```python
from build123d import *

# Parameters (mm, degrees)
SKETCH1_R              = 5.08
BOSS_EXTRUDE1_DEPTH    = 6.35
F_10_32_TAPPED_HOLE1_D = 4.826
SKETCH7_R              = 8.73125
CUT_EXTRUDE1_DEPTH     = 7.35
SKETCH8_R              = 6.35
CUT_EXTRUDE2_DEPTH     = 7.35
FILLET1_R              = 25.4
FILLET2_R              = 6.35
F_4_40_TAPPED_HOLE1_D  = 2.2606


with BuildPart() as part:
    # Sketch1 → Boss-Extrude1 (new body)
    with BuildSketch(Plane(origin=(0, 0, 0), x_dir=(1, 0, 0), z_dir=(0, 1, 0))):
        with Locations((0, -15.08125)):
            Circle(SKETCH1_R)
        with BuildLine():
            Line((1.984375, -15.750488274), (-48.417187476, -22.100488274))
            ThreePointArc((-48.417187476, -22.100488274), (-66.152050749, -8.334375), (-52.385937476, 9.400488274))
            Line((-52.385937476, 9.400488274), (-1.984375, 15.750488274))
            ThreePointArc((-1.984375, 15.750488274), (15.750488274, 1.984375), (1.984375, -15.750488274))
        make_face()
        with BuildLine():
            Line((1.984375, 15.750488274), (52.385937476, 9.400488274))
            ThreePointArc((52.385937476, 9.400488274), (66.152050749, -8.334375), (48.417187476, -22.100488274))
            Line((48.417187476, -22.100488274), (-1.984375, -15.750488274))
            ThreePointArc((-1.984375, -15.750488274), (-15.750488274, 1.984375), (1.984375, 15.750488274))
        make_face()
    extrude(amount=BOSS_EXTRUDE1_DEPTH)

    # #10-32 Tapped Hole1 (through all)
    with Locations(Plane(origin=(0, 6.35, 0), x_dir=(1, 0, 0), z_dir=(0, 1, 0))):
        with Locations((-50.401562476, -6.35), (50.401562476, -6.35)):
            Hole(F_10_32_TAPPED_HOLE1_D / 2)

    # Sketch7 → Cut-Extrude1 (cut, through all)
    with BuildSketch(Plane(origin=(0, 6.35, 0), x_dir=(1, 0, 0), z_dir=(0, 1, 0))):
        Circle(SKETCH7_R)
    extrude(amount=-CUT_EXTRUDE1_DEPTH, mode=Mode.SUBTRACT)

    # Sketch8 → Cut-Extrude2 (cut, through all)
    with BuildSketch(Plane(origin=(0, 6.35, 0), x_dir=(1, 0, 0), z_dir=(0, 1, 0))):
        with Locations((-38.1, 12.7)):
            Circle(SKETCH8_R)
        with Locations((38.1, 12.7)):
            Circle(SKETCH8_R)
    extrude(amount=-CUT_EXTRUDE2_DEPTH, mode=Mode.SUBTRACT)

    # Fillet1
    fillet1_edges = [part.edges().sort_by_distance(p)[0] for p in [
        (-4.844257487, 3.175, 16.6108151),
        (4.844257487, 3.175, 16.6108151),
    ]]
    fillet(fillet1_edges, radius=FILLET1_R)

    # Fillet2
    fillet2_edges = [part.edges().sort_by_distance(p)[0] for p in [
        (-31.789208912, 3.175, -11.995432159),
        (-44.038818433, 3.175, -10.452126424),
        (31.789208912, 3.175, -11.995432159),
        (44.038818433, 3.175, -10.452126424),
    ]]
    fillet(fillet2_edges, radius=FILLET2_R)

    # #4-40 Tapped Hole1 (through all)
    with Locations(Plane(origin=(0, 6.35, 0), x_dir=(1, 0, 0), z_dir=(0, 1, 0))):
        with Locations((-15.08125, 0), (15.08125, 0), (0, -15.08125)):
            Hole(F_4_40_TAPPED_HOLE1_D / 2)


solid = part.part
```
Read the model definition and answer for the solid it produces. Units are mm, in the model's axes. A direction names the side the tool comes from. Coordinates: 2 decimals unless noted, no trailing zeros. Loops run counter-clockwise (first coordinate to the right, second up) from the corner with the lowest first, then second, coordinate; pieces in that order, holes last.
(1) A tool of negligible diameter and unlimited length cuts with its end or side. For faces 1 (the face through (-31.551, 3.131, 19.976)), 2 (the face through (-47.99, 3.13, 6.24)), from which of +Z, -Z, +X, -X, +Y, -Y can it reach the whole face along a straight path? Write none if from no direction.
Solution:
face 1: +Z, +Y, -Y
face 2: +Y, -Y
(2) The part is cut by section D-D (z = 6.35). Determine the outline of the cut face in (x, y), and give its area (3 significant figures).
Solution:
outline: (-66.28, 0) - (-52.81, 0) - (-52.81, 6.35) - (-66.28, 6.35) - close; (-47.99, 0) - (-5.99, 0) - (-5.99, 6.35) - (-47.99, 6.35) - close; (5.99, 0) - (47.99, 0) - (47.99, 6.35) - (5.99, 6.35) - close; (52.81, 0) - (66.28, 0) - (66.28, 6.35) - (52.81, 6.35) - close
area: 704 mm2
(3) The mould has two halves that part along Z. Classify faces 3 (the face through (-66.1, 3.1, 8.7)), 4 (the face through (32.017, 3.131, 20.034)), 5 (the face through (14.037, 3.131, 0.433)): released by +Z, released by -Z, zero draft, split by the parting line, or undercut.
Solution:
face 3: split by the parting line
face 4: released by +Z
face 5: undercut
(4) The part is cut by section B-B (z = -2.5). Determine the outline of the cut face in (x, y), and give its area (3 significant figures).
Solution:
outline: (-63.58, 0) - (-8.37, 0) - (-8.37, 6.35) - (-63.58, 6.35) - close; (8.37, 0) - (63.58, 0) - (63.58, 6.35) - (8.37, 6.35) - close
area: 701 mm2
(5) Consider line 1 along Z through (x, y) = (0, 3) (3 decimals); line 2 along X through (y, z) = (6.25, 5); line 3 along X through (y, z) = (3.5, -8). Determine where each line is inside the solid, lowest interval first.
Solution:
line 1: z = -15.875 to -8.731, 8.731 to 13.951, 16.212 to 20.161
line 2: x = -66.22 to -52.4, -48.4 to -7.16, 7.16 to 48.4, 52.4 to 66.22
line 3: x = -57.19 to -42.37, -33.83 to -3.5, 3.5 to 33.83, 42.37 to 57.19
(6) Flat-ended cylindrical pins translate along their axes: pin 1 Ø4 at (x, z) = (-50.4, 6.35) entering from -Y; pin 2 Ø3 at (y, z) = (2, 16.5) entering from -X; pin 3 Ø3 at (y, z) = (4, 3.5) entering from +X. Find the tip coordinate at first contact, or state that the pin passes through.
Solution:
pin 1: passes through
pin 2: stops at x = -63.71
pin 3: stops at x = 66.22
(7) The part is cut by section A-A (x = 0). Determine the outline of the cut face in (y, z) (3 decimals), and give its area (3 significant figures).
Solution:
outline: (0, -15.875) - (6.35, -15.875) - (6.35, -8.731) - (0, -8.731) - close; (0, 8.731) - (6.35, 8.731) - (6.35, 13.951) - (0, 13.951) - close; (0, 16.212) - (6.35, 16.212) - (6.35, 20.161) - (0, 20.161) - close
area: 104 mm2
(8) The part is cut by section C-C (y = 3.5). Count the separate pieces of the cut face and the enclosed holes in it, and give its area (3 significant figures).
Solution:
separate pieces: 1
enclosed holes: 6
area: 3,680 mm2
